Check sheet for the modelled part. Datum: model origin and axes. Units: mm. Face numbers are marked on the shaded views. A direction names the side the tool comes from. Coordinates: 2 decimals unless noted, no trailing zeros. Answer as CSV lines item,"result".
from build123d import *

# Parameters (mm, degrees)
SKETCH1_W           = 63.5
SKETCH1_H           = 63.5
BOSS_EXTRUDE1_DEPTH = 704.85
SKETCH2_W           = 57.15
SKETCH2_H           = 57.15
CUT_EXTRUDE1_DEPTH  = 705.85
CUT_EXTRUDE2_REACH  = 65.5
SKETCH3_R           = 17.4625
SKETCH8_R           = 2.15265
CUT_EXTRUDE6_DEPTH  = 64.5
SKETCH10_R          = 2.15265
CUT_EXTRUDE7_DEPTH  = 64.5
CUT_EXTRUDE9_REACH  = 65.5
SKETCH13_R          = 16
SKETCH14_R          = 2.625
SKETCH14_R_2        = 16
CUT_EXTRUDE10_DEPTH = 3.175
CUT_EXTRUDE11_START = -3.175
CUT_EXTRUDE11_DEPTH = 3.175
CUT_EXTRUDE13_REACH = 65.5
SKETCH17_W          = 19.05
SKETCH17_H          = 25.4


with BuildPart() as part:
    # Sketch1 → Boss-Extrude1 (new body)
    with BuildSketch(Plane(origin=(0, 0, 0), x_dir=(0, 0, -1), z_dir=(1, 0, 0))):
        Rectangle(SKETCH1_W, SKETCH1_H)
    extrude(amount=BOSS_EXTRUDE1_DEPTH)

    # Sketch2 → Cut-Extrude1 (cut, through all)
    with BuildSketch(Plane(origin=(704.85, 0, 0), x_dir=(0, 0, -1), z_dir=(1, 0, 0))):
        Rectangle(SKETCH2_W, SKETCH2_H)
    extrude(amount=-CUT_EXTRUDE1_DEPTH, mode=Mode.SUBTRACT)

    # Sketch3 → Cut-Extrude2 (cut, up to next)
    with BuildSketch(Plane.XY.offset(31.75), mode=Mode.PRIVATE) as cut_extrude2_sk1:
        with Locations((352.425, 0)):
            Circle(SKETCH3_R)
    cut_extrude2_tool1 = extrude(cut_extrude2_sk1.sketch, amount=-CUT_EXTRUDE2_REACH, mode=Mode.PRIVATE) & part.part
    add(cut_extrude2_tool1.solids().sort_by_distance((352.425, 0, 31.75))[0], mode=Mode.SUBTRACT)
    # Sketch3 → Cut-Extrude2 (cut, up to next)
    with BuildSketch(Plane.XY.offset(31.75), mode=Mode.PRIVATE) as cut_extrude2_sk2:
        with Locations((34.925, 0)):
            Circle(SKETCH3_R)
    cut_extrude2_tool2 = extrude(cut_extrude2_sk2.sketch, amount=-CUT_EXTRUDE2_REACH, mode=Mode.PRIVATE) & part.part
    add(cut_extrude2_tool2.solids().sort_by_distance((34.925, 0, 31.75))[0], mode=Mode.SUBTRACT)
    # Sketch3 → Cut-Extrude2 (cut, up to next)
    with BuildSketch(Plane.XY.offset(31.75), mode=Mode.PRIVATE) as cut_extrude2_sk3:
        with Locations((669.925, 0)):
            Circle(SKETCH3_R)
    cut_extrude2_tool3 = extrude(cut_extrude2_sk3.sketch, amount=-CUT_EXTRUDE2_REACH, mode=Mode.PRIVATE) & part.part
    add(cut_extrude2_tool3.solids().sort_by_distance((669.925, 0, 31.75))[0], mode=Mode.SUBTRACT)

    # Sketch8 → Cut-Extrude6 (cut, through all)
    with BuildSketch(Plane(origin=(0, 31.75, 0), x_dir=(1, 0, 0), z_dir=(0, 1, 0))):
        with Locations((466.725, 0)):
            Circle(SKETCH8_R)
        with Locations((123.825, 0)):
            Circle(SKETCH8_R)
        with Locations((581.025, 0)):
            Circle(SKETCH8_R)
        with Locations((238.125, 0)):
            Circle(SKETCH8_R)
    extrude(amount=-CUT_EXTRUDE6_DEPTH, mode=Mode.SUBTRACT)

    # Sketch10 → Cut-Extrude7 (cut, through all)
    with BuildSketch(Plane.XY.offset(31.75)):
        with Locations((225.425, 0)):
            Circle(SKETCH10_R)
        with Locations((568.325, 0)):
            Circle(SKETCH10_R)
        with Locations((136.525, 0)):
            Circle(SKETCH10_R)
        with Locations((479.425, 0)):
            Circle(SKETCH10_R)
    extrude(amount=-CUT_EXTRUDE7_DEPTH, mode=Mode.SUBTRACT)

    # Sketch13 → Cut-Extrude9 (cut, up to next)
    with BuildSketch(Plane(origin=(0, 0, -31.75), x_dir=(-1, 0, 0), z_dir=(0, 0, -1)), mode=Mode.PRIVATE) as cut_extrude9_sk1:
        with Locations((-352.425, 0)):
            Circle(SKETCH13_R)
    cut_extrude9_tool1 = extrude(cut_extrude9_sk1.sketch, amount=-CUT_EXTRUDE9_REACH, mode=Mode.PRIVATE) & part.part
    add(cut_extrude9_tool1.solids().sort_by_distance((352.425, 0, -31.75))[0], mode=Mode.SUBTRACT)
    # Sketch13 → Cut-Extrude9 (cut, up to next)
    with BuildSketch(Plane(origin=(0, 0, -31.75), x_dir=(-1, 0, 0), z_dir=(0, 0, -1)), mode=Mode.PRIVATE) as cut_extrude9_sk2:
        with Locations((-34.925, 0)):
            Circle(SKETCH13_R)
    cut_extrude9_tool2 = extrude(cut_extrude9_sk2.sketch, amount=-CUT_EXTRUDE9_REACH, mode=Mode.PRIVATE) & part.part
    add(cut_extrude9_tool2.solids().sort_by_distance((34.925, 0, -31.75))[0], mode=Mode.SUBTRACT)
    # Sketch13 → Cut-Extrude9 (cut, up to next)
    with BuildSketch(Plane(origin=(0, 0, -31.75), x_dir=(-1, 0, 0), z_dir=(0, 0, -1)), mode=Mode.PRIVATE) as cut_extrude9_sk3:
        with Locations((-669.925, 0)):
            Circle(SKETCH13_R)
    cut_extrude9_tool3 = extrude(cut_extrude9_sk3.sketch, amount=-CUT_EXTRUDE9_REACH, mode=Mode.PRIVATE) & part.part
    add(cut_extrude9_tool3.solids().sort_by_distance((669.925, 0, -31.75))[0], mode=Mode.SUBTRACT)

    # Sketch14 → Cut-Extrude10 (cut)
    with BuildSketch(Plane(origin=(0, 0, -31.75), x_dir=(-1, 0, 0), z_dir=(0, 0, -1))):
        with Locations((-655.782864376, 14.142135624)):
            Circle(SKETCH14_R)
        with Locations((-338.282864376, 14.142135624)):
            Circle(SKETCH14_R)
        with Locations((-20.782864376, 14.142135624)):
            Circle(SKETCH14_R)
        with Locations((-352.425, 0)):
            Circle(SKETCH14_R_2)
        with Locations((-34.925, 0)):
            Circle(SKETCH14_R_2)
        with Locations((-669.925, 0)):
            Circle(SKETCH14_R_2)
        with Locations((-338.282864376, -14.142135624)):
            Circle(SKETCH14_R)
        with Locations((-366.567135624, -14.142135624)):
            Circle(SKETCH14_R)
        with Locations((-366.567135624, 14.142135624)):
            Circle(SKETCH14_R)
        with Locations((-20.782864376, -14.142135624)):
            Circle(SKETCH14_R)
        with Locations((-49.067135624, -14.142135624)):
            Circle(SKETCH14_R)
        with Locations((-49.067135624, 14.142135624)):
            Circle(SKETCH14_R)
        with Locations((-655.782864376, -14.142135624)):
            Circle(SKETCH14_R)
        with Locations((-684.067135624, -14.142135624)):
            Circle(SKETCH14_R)
        with Locations((-684.067135624, 14.142135624)):
            Circle(SKETCH14_R)
    extrude(amount=-CUT_EXTRUDE10_DEPTH, mode=Mode.SUBTRACT)

    # Sketch15 → Cut-Extrude11 (cut)
    with BuildSketch(Plane.XY.offset(31.75).offset(CUT_EXTRUDE11_START)):
        with BuildLine():
            Line((364.710980323, -15.998290924), (362.776389114, -14.063699715))
            ThreePointArc((362.776389114, -14.063699715), (352.425, -17.4625), (342.073610886, -14.063699715))
            Line((342.073610886, -14.063699715), (340.139019677, -15.998290924))
            ThreePointArc((340.139019677, -15.998290924), (336.426709076, -15.998290924), (336.426709076, -12.285980323))
            Line((336.426709076, -12.285980323), (338.361300285, -10.351389114))
            ThreePointArc((338.361300285, -10.351389114), (334.9625, 0), (338.361300285, 10.351389114))
            Line((338.361300285, 10.351389114), (336.426709076, 12.285980323))
            ThreePointArc((336.426709076, 12.285980323), (336.426709076, 15.998290924), (340.139019677, 15.998290924))
            Line((340.139019677, 15.998290924), (342.073610886, 14.063699715))
            ThreePointArc((342.073610886, 14.063699715), (352.425, 17.4625), (362.776389114, 14.063699715))
            Line((362.776389114, 14.063699715), (364.710980323, 15.998290924))
            ThreePointArc((364.710980323, 15.998290924), (368.423290924, 15.998290924), (368.423290924, 12.285980323))
            Line((368.423290924, 12.285980323), (366.488699715, 10.351389114))
            ThreePointArc((366.488699715, 10.351389114), (369.8875, 0), (366.488699715, -10.351389114))
            Line((366.488699715, -10.351389114), (368.423290924, -12.285980323))
            ThreePointArc((368.423290924, -12.285980323), (368.423290924, -15.998290924), (364.710980323, -15.998290924))
        make_face()
        with BuildLine():
            Line((50.923290924, 12.285980323), (48.988699715, 10.351389114))
            ThreePointArc((48.988699715, 10.351389114), (52.3875, 0), (48.988699715, -10.351389114))
            Line((48.988699715, -10.351389114), (50.923290924, -12.285980323))
            ThreePointArc((50.923290924, -12.285980323), (50.923290924, -15.998290924), (47.210980323, -15.998290924))
            Line((47.210980323, -15.998290924), (45.276389114, -14.063699715))
            ThreePointArc((45.276389114, -14.063699715), (34.925, -17.4625), (24.573610886, -14.063699715))
            Line((24.573610886, -14.063699715), (22.639019677, -15.998290924))
            ThreePointArc((22.639019677, -15.998290924), (18.926709076, -15.998290924), (18.926709076, -12.285980323))
            Line((18.926709076, -12.285980323), (20.861300285, -10.351389114))
            ThreePointArc((20.861300285, -10.351389114), (17.4625, 0), (20.861300285, 10.351389114))
            Line((20.861300285, 10.351389114), (18.926709076, 12.285980323))
            ThreePointArc((18.926709076, 12.285980323), (18.926709076, 15.998290924), (22.639019677, 15.998290924))
            Line((22.639019677, 15.998290924), (24.573610886, 14.063699715))
            ThreePointArc((24.573610886, 14.063699715), (34.925, 17.4625), (45.276389114, 14.063699715))
            Line((45.276389114, 14.063699715), (47.210980323, 15.998290924))
            ThreePointArc((47.210980323, 15.998290924), (50.923290924, 15.998290924), (50.923290924, 12.285980323))
        make_face()
        with BuildLine():
            Line((685.923290924, 12.285980323), (683.988699715, 10.351389114))
            ThreePointArc((683.988699715, 10.351389114), (687.3875, 0), (683.988699715, -10.351389114))
            Line((683.988699715, -10.351389114), (685.923290924, -12.285980323))
            ThreePointArc((685.923290924, -12.285980323), (685.923290924, -15.998290924), (682.210980323, -15.998290924))
            Line((682.210980323, -15.998290924), (680.276389114, -14.063699715))
            ThreePointArc((680.276389114, -14.063699715), (669.925, -17.4625), (659.573610886, -14.063699715))
            Line((659.573610886, -14.063699715), (657.639019677, -15.998290924))
            ThreePointArc((657.639019677, -15.998290924), (653.926709076, -15.998290924), (653.926709076, -12.285980323))
            Line((653.926709076, -12.285980323), (655.861300285, -10.351389114))
            ThreePointArc((655.861300285, -10.351389114), (652.4625, 0), (655.861300285, 10.351389114))
            Line((655.861300285, 10.351389114), (653.926709076, 12.285980323))
            ThreePointArc((653.926709076, 12.285980323), (653.926709076, 15.998290924), (657.639019677, 15.998290924))
            Line((657.639019677, 15.998290924), (659.573610886, 14.063699715))
            ThreePointArc((659.573610886, 14.063699715), (669.925, 17.4625), (680.276389114, 14.063699715))
            Line((680.276389114, 14.063699715), (682.210980323, 15.998290924))
            ThreePointArc((682.210980323, 15.998290924), (685.923290924, 15.998290924), (685.923290924, 12.285980323))
        make_face()
    extrude(amount=CUT_EXTRUDE11_DEPTH, mode=Mode.SUBTRACT)

    # Sketch17 → Cut-Extrude13 (cut, up to next)
    with BuildSketch(Plane.XZ.offset(31.75), mode=Mode.PRIVATE) as cut_extrude13_sk1:
        with Locations((352.425, -12.7)):
            Rectangle(SKETCH17_W, SKETCH17_H)
    cut_extrude13_tool1 = extrude(cut_extrude13_sk1.sketch, amount=-CUT_EXTRUDE13_REACH, mode=Mode.PRIVATE) & part.part
    add(cut_extrude13_tool1.solids().sort_by_distance((352.425, -31.75, -12.7))[0], mode=Mode.SUBTRACT)


solid = part.part
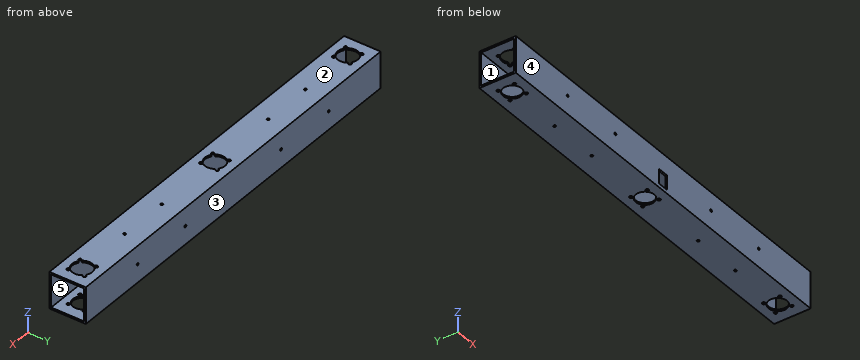
1) Mould release check, pull along Y, two halves, no side actions. Record for the marked faces 1, 2 and 3: pulls with the +Y half, pulls with the -Y half, needs draft (parallel to the pull), parting line crosses it, or undercut.
Answer key:
face 1,"undercut"
face 2,"needs draft"
face 3,"pulls with the +Y half"
2) Thickness scan on line 1 along X through (y, z) = (30, 0); line 2 along Z through (x, y) = (369, 11) (3 decimals). Record the ranges inside material, lowest first.
Answer key:
line 1,"x = 0 to 121.67, 125.98 to 235.97, 240.28 to 464.57, 468.88 to 578.87, 583.18 to 704.85"
line 2,"z = -31.75 to -28.575, 28.575 to 31.75"
3) Depth check by flat-ended pin: P1, Ø4, axis at x = 366.57, y = 14.14, coming from the +Z side; P2, Ø8.5, axis at x = 684.07, y = 14.14, coming from the +Z side. Enter the tip coordinate at first touch or a pass-through.
Answer key:
P1,"passes through"
P2,"stops at z = 31.75"
4) Tool access check on the marked faces 4 and 5. Record the directions out of +Z, -Z, +X, -X, +Y, -Y that give a thin tool (end or side, any length) a straight path to the whole face; none if there is none.
Answer key:
face 4,"+Z, -Z, +X, -X, -Y"
face 5,"+X, -X"
